Verification items for the finished model (mm, model axes). A direction names the side the tool comes from. Give positions to 0.01 mm unless a question says otherwise; leave off trailing zeros. Write each loop counter-clockwise with the first axis right and the second up, starting at its lowest first coordinate (ties: lowest second). Pieces come first, ordered by that corner, then holes.
from build123d import *

# Parameters (mm, degrees)
BOSS_EXTRUDE2_DEPTH = 40
SKETCH2_5_W         = 20
SKETCH2_5_H         = 20
BOSS_EXTRUDE3_DEPTH = 10


with BuildPart() as part:
    # Sketch2 → Boss-Extrude2 (new body)
    with BuildSketch(Plane.XY):
        Polygon((30, 20.406682394), (10, 40.406682394), (10, 20.406682394), (-10, 20.406682394), (-10, 40.406682394), (-30, 20.406682394), (-30, -40.406682394), (30, -40.406682394), align=None)
    extrude(amount=BOSS_EXTRUDE2_DEPTH)

    # Sketch2_5 → Boss-Extrude3 (add)
    with BuildSketch(Plane.XY):
        Polygon((-30, 20.406682394), (-10, 40.406682394), (-30, 40.406682394), align=None)
        with Locations((0, 30.406682394)):
            Rectangle(SKETCH2_5_W, SKETCH2_5_H)
        Polygon((30, 40.406682394), (10, 40.406682394), (30, 20.406682394), align=None)
    extrude(amount=BOSS_EXTRUDE3_DEPTH)

    # Mirror1: part across plane


with BuildPart() as part_1:
    add(part.part)
    add(part.part.mirror(Plane.XY.offset(40)))


solid = part_1.part
Item 1: Sectioned sample at C-C on x = 5. Record the cut outline in (y, z), then the cut area to 3 significant figures.
Answer key:
outline: (-40.41, 0) - (40.41, 0) - (40.41, 10) - (20.41, 10) - (20.41, 70) - (40.41, 70) - (40.41, 80) - (-40.41, 80) - close
area: 5,270 mm2
Item 2: Sectioned sample at B-B on y = 25. Record the cut outline in (x, z).
Answer key:
outline: (-30, 0) - (30, 0) - (30, 10) - (25.41, 10) - (25.41, 70) - (30, 70) - (30, 80) - (-30, 80) - (-30, 70) - (-25.41, 70) - (-25.41, 10) - (-30, 10) - close; hole (-10, 10) - (10, 10) - (10, 70) - (-10, 70) - close
Item 3: Release check for a two-part mould opening along Z. For faces 4 (the face through (0, 1, 0)), 5 (the face through (0, 31, 10)), 6 (the face through (0, 1, 80)) record: released by +Z, released by -Z, zero draft, split by the parting line, or undercut.
Answer key:
face 4: released by -Z
face 5: undercut
face 6: released by +Z
Item 4: Set-up check for faces 1 (the face through (0, 31, 70)), 2 (the face through (20.14, 30.267, 40.42)), 3 (the face through (-19.86, 30.547, 40.42)): record each of +Z, -Z, +X, -X, +Y, -Y from which the full face is reachable in a straight line by a thin tool's end or side.
Answer key:
face 1: +Y
face 2: +X, +Y
face 3: -X, +Y
Item 5: Depth check by flat-ended pin: pin 1 (6 mm diameter, centred on y = 27, z = 49.5, fed in from +X); pin 2 (10 mm diameter, centred on x = -16, y = 30, fed in from -Z); pin 3 (6 mm diameter, centred on x = -3.5, z = 34, fed in from +Y); pin 4 (2 mm diameter, centred on x = -19.5, z = 43, fed in from +Y). Enter the tip coordinate at first touch or a pass-through.
Answer key:
pin 1: stops at x = 26.41
pin 2: stops at z = 0
pin 3: stops at y = 20.41
pin 4: stops at y = 31.91
Item 6: Sectioned sample at A-A on z = 51.5. Record the cut outline in (x, y).
Answer key:
outline: (-30, -40.41) - (30, -40.41) - (30, 20.41) - (10, 40.41) - (10, 20.41) - (-10, 20.41) - (-10, 40.41) - (-30, 20.41) - close
Item 7: Scan lines: line 1 along Y through (x, z) = (-9, 45.5); line 2 along X through (y, z) = (22, 62); line 3 along Y through (x, z) = (16, 20.5). Record each from-to range of solid material in increasing order.
Answer key:
line 1: y = -40.41 to 20.41
line 2: x = -28.41 to -10, 10 to 28.41
line 3: y = -40.41 to 34.41
